Design review of the part shown in the three views and the two pictorial views. Dimensions are in mm from the part's minimum x, y and z. A direction names the side the tool comes from. Give positions to 0.01 mm unless a question says otherwise; leave off trailing zeros. Loops run counter-clockwise (first coordinate to the right, second up) from the corner with the lowest first, then second, coordinate; pieces in that order, holes last.
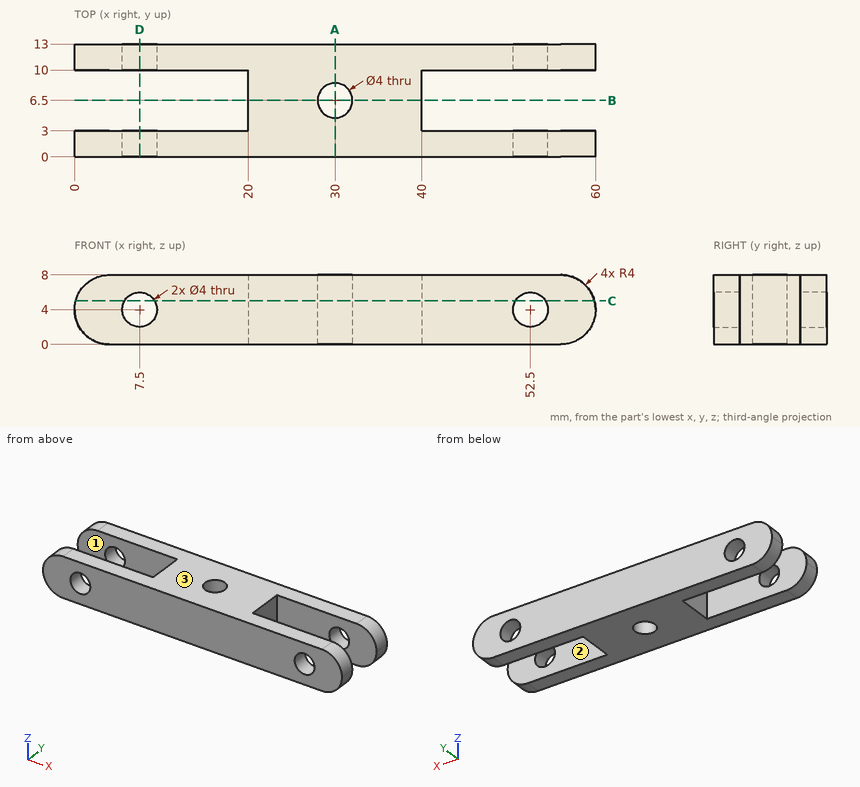
Q1. Machinability: for the marked faces 1, 2 and 3, which of the approach directions +Z, -Z, +X, -X, +Y, -Y give a long, thin tool a straight path to every point of the face, cutting with its end or side? Answer none if there is none.
Answers:
face 1: +Z, -Z, -X
face 2: +Z, -Z, +X
face 3: +Z, +X, -X, +Y, -Y
Q2. For pin 1 Ø2.5 at (x, z) = (52.5, 4) entering from -Y; pin 2 Ø3.5 at (y, z) = (5.5, 3.5) entering from -X; pin 3 Ø1 at (y, z) = (4.5, 5) entering from +X, all flat-tipped, find the tip position at first contact; note any pin that passes through.
Answers:
pin 1: passes through
pin 2: stops at x = 20
pin 3: stops at x = 40
Q3. Consider section C-C on z = 5. Count the separate pieces of the cut face and the enclosed holes in it, plus the area to 3 significant figures.
Answers:
separate pieces: 5
enclosed holes: 1
area: 444 mm2
Q4. Consider section A-A on x = 30. Give the boundary of the cut face in (y, z), plus the area to 3 significant figures.
Answers:
outline: (0, 0) - (4.5, 0) - (4.5, 8) - (0, 8) - close; (8.5, 0) - (13, 0) - (13, 8) - (8.5, 8) - close
area: 72.0 mm2
Q5. For probe 1 along X at (y, z) = (10.9, 4); probe 2 along Y at (x, z) = (51, 6.75); probe 3 along X at (y, z) = (9.25, 2.25), list the stretches that pass through material, from the lowest coordinate up.
Answers:
probe 1: x = 0 to 5.5, 9.5 to 50.5, 54.5 to 60
probe 2: y = 0 to 3, 10 to 13
probe 3: x = 20 to 40
Q6. Consider section D-D on x = 7.5. Give the boundary of the cut face in (y, z).
Answers:
outline: (0, 0) - (3, 0) - (3, 2) - (0, 2) - close; (0, 6) - (3, 6) - (3, 8) - (0, 8) - close; (10, 0) - (13, 0) - (13, 2) - (10, 2) - close; (10, 6) - (13, 6) - (13, 8) - (10, 8) - close
Q7. Consider section B-B on y = 6.5. Give the boundary of the cut face in (x, z).
Answers:
outline: (20, 0) - (28, 0) - (28, 8) - (20, 8) - close; (32, 0) - (40, 0) - (40, 8) - (32, 8) - close
